from build123d import *

# Parameters (mm, degrees)
SKETCH001_W = 142.252221
SKETCH001_H = 119.938137
PAD_DEPTH   = 25


with BuildPart() as pad:
    # Sketch001 → Pad (new body)
    with BuildSketch(Plane.YZ):
        with Locations((-0.633922, -1.648195)):
            Rectangle(SKETCH001_W, SKETCH001_H)
    extrude(amount=PAD_DEPTH)


with BuildPart() as cut:
    # Sketch → Revolution (revolve)
    with BuildSketch(Plane.XY):
        Polygon((0, 0), (0, 50), (50, 0), align=None)
    revolve(axis=Axis((0, 0, 0), (1, 0, 0)))

    # Cut: cut Pad
    add(pad.part, mode=Mode.SUBTRACT)


solid = cut.part
Input: part model. Units: mm. Frame: model coordinates. Coordinates: 2 decimals unless noted, no trailing zeros. Loops run counter-clockwise (first coordinate to the right, second up) from the corner with the lowest first, then second, coordinate; pieces in that order, holes last.
(1) First-contact query: pin 1 Ø1.5 at (x, y) = (29, -13) entering from +Z; pin 2 Ø1 at (y, z) = (3.5, 5.5) entering from +X; pin 3 Ø1.5 at (y, z) = (-4, -9) entering from +X. Flat tips, straight axial feed; report the tip coordinate or a pass-through.
(2) Material intervals for probe 1 along Z at (x, y) = (29.75, 17.5); probe 2 along Y at (x, z) = (37.75, -1), sorted ascending.
(3) Section A-A on x = 42.75. Return the cut outline in (y, z), then the cut area to 3 significant figures.
(4) Section B-B on x = 36. Return the cut outline in (y, z), then the cut area to 3 significant figures.
Data:
1. pin 1: stops at z = 17.59
1. pin 2: stops at x = 43.98
1. pin 3: stops at x = 40.9
2. probe 1: z = -10.19 to 10.19
2. probe 2: y = -12.21 to 12.21
3. outline: circle Ø14.5 at (0, 0)
3. area: 165 mm2
4. outline: circle Ø28 at (0, 0)
4. area: 616 mm2
